```python
from build123d import *

# Parameters (mm, degrees)
CROQUIS1_W              = 139.5
CROQUIS1_H              = 25
SALIENTE_EXTRUIR1_DEPTH = 10.1
CORTAR_EXTRUIR1_DEPTH   = 26
CROQUIS3_R              = 2.675
CORTAR_EXTRUIR2_DEPTH   = 15
CORTAR_EXTRUIR3_DEPTH   = 11.1
CORTAR_EXTRUIR4_DEPTH   = 5.5
CROQUIS7_R              = 2.8
CORTAR_EXTRUIR5_DEPTH   = 15


with BuildPart() as part:
    # Croquis1 → Saliente-Extruir1 (new body)
    with BuildSketch(Plane(origin=(0, 0, 0), x_dir=(1, 0, 0), z_dir=(0, 1, 0))):
        Rectangle(CROQUIS1_W, CROQUIS1_H)
    extrude(amount=SALIENTE_EXTRUIR1_DEPTH)

    # Croquis2 → Cortar-Extruir1 (cut, through all)
    with BuildSketch(Plane.XY.offset(12.5)):
        Polygon((-69.75, 10.1), (-69.75, 0), (-52.25, 0), (-52.25, 1.4), (-68.35, 1.4), (-68.35, 10.1), align=None)
    extrude(amount=-CORTAR_EXTRUIR1_DEPTH, mode=Mode.SUBTRACT)

    # Croquis3 → Cortar-Extruir2 (cut)
    with BuildSketch(Plane.ZY.offset(68.35)):
        with Locations((-7.5, 5.75)):
            Circle(CROQUIS3_R)
        with Locations((7.5, 5.75)):
            Circle(CROQUIS3_R)
    extrude(amount=-CORTAR_EXTRUIR2_DEPTH, mode=Mode.SUBTRACT)

    # Croquis4 → Cortar-Extruir3 (cut, through all)
    with BuildSketch(Plane(origin=(0, 10.1, 0), x_dir=(1, 0, 0), z_dir=(0, 1, 0))):
        with BuildLine():
            Line((49.75, 1.575), (61.75, 1.575))
            ThreePointArc((61.75, 1.575), (63.325, 0), (61.75, -1.575))
            Line((61.75, -1.575), (49.75, -1.575))
            ThreePointArc((49.75, -1.575), (48.175, 0), (49.75, 1.575))
        make_face()
    extrude(amount=-CORTAR_EXTRUIR3_DEPTH, mode=Mode.SUBTRACT)

    # Croquis5 → Cortar-Extruir4 (cut)
    with BuildSketch(Plane.XZ):
        with BuildLine():
            Line((49.75, 4.325), (61.75, 4.325))
            ThreePointArc((61.75, 4.325), (66.075, 0), (61.75, -4.325))
            Line((61.75, -4.325), (49.75, -4.325))
            ThreePointArc((49.75, -4.325), (45.425, 0), (49.75, 4.325))
        make_face()
    extrude(amount=-CORTAR_EXTRUIR4_DEPTH, mode=Mode.SUBTRACT)

    # Croquis7 → Cortar-Extruir5 (cut)
    with BuildSketch(Plane(origin=(69.75, 0, 0), x_dir=(0, 0, -1), z_dir=(1, 0, 0))):
        with Locations((-8.4125, 5.05)):
            Circle(CROQUIS7_R)
        with Locations((8.4125, 5.05)):
            Circle(CROQUIS7_R)
    extrude(amount=-CORTAR_EXTRUIR5_DEPTH, mode=Mode.SUBTRACT)


solid = part.part
```
Source: CAD feature listing. Evaluate the final solid. Frame: model axes, mm. A direction names the side the tool comes from. Coordinates: 2 decimals unless noted, no trailing zeros. Write each loop counter-clockwise with the first axis right and the second up, starting at its lowest first coordinate (ties: lowest second). Pieces come first, ordered by that corner, then holes. Notation, with made-up numbers: (-32.75, 64) -> (-28.75, 64) arc R13 ccw to (-28.75, 69) -> close; hole circle Ø10 at (-0.75, -23). An arc over 180 degrees is marked (long way). Return JSON: item names as keys, results as strings. Group by question number.
1) Section query A-A, the plane z = 7.5. Return loops of the section in (x, y) (3 decimals), plus the area to 3 significant figures.
2) Ray query, line 1 along Y through (x, z) = (-60, 7.5) (3 decimals); line 2 along X through (y, z) = (8.25, 0) (3 decimals); line 3 along Y through (x, z) = (-55.5, -1.5). Return the intervals inside material, ascending.
3) Set-up query: faces 1 (the face through (-60.96, 4.12, -9.62)), 2 (the face through (62.355, 5.173, -5.615)), 3 (the face through (56, 3, 4.325)). Return all of +Z, -Z, +X, -X, +Y, -Y with unobstructed straight access to the full face (end or side cutting, diameter ignored); none if empty.
4) Contact query for flat-ended pins moving along their axis: P1, Ø1.6, axis at y = 6, z = -6, coming from the -X side; P2, Ø5, axis at x = -58, z = 6, coming from the -Y side; P3, Ø2.5, axis at x = 58, z = -2, coming from the -Y side. Output: stop coordinate, or through.
5) Mould query, pull axis Y, two halves, no side actions, for faces 4 (the face through (62.355, 3.978, 5.826)), 5 (the face through (66.074, 2.712, 0.095)), 6 (the face through (56, 5.5, -2)). Classes: +Y half, -Y half, draft (parallel to the pull), parting line (faces both ways), or undercut.
From the geometry:
{
 "1": {"outline": "(-68.35, 1.4) -> (-52.25, 1.4) -> (-52.25, 0) -> (69.75, 0) -> (69.75, 2.403) -> (54.75, 2.403) -> (54.75, 7.697) -> (69.75, 7.697) -> (69.75, 10.1) -> (-68.35, 10.1) -> (-68.35, 8.425) -> (-53.35, 8.425) -> (-53.35, 3.075) -> (-68.35, 3.075) -> close", "area": "1,210 mm²"},
 "2": {"line 1": "1.4 to 3.075, 8.425 to 10.1", "line 2": "-68.35 to 48.175, 63.325 to 69.75", "line 3": "1.4 to 10.1"},
 "3": {"face 1": "-X", "face 2": "+X", "face 3": "-Y"},
 "4": {"P1": "x = -53.35", "P2": "y = 1.4", "P3": "y = 5.5"},
 "5": {"face 4": "undercut", "face 5": "draft", "face 6": "-Y half"}
}
